Here's how the part is built. I have some questions about the finished solid (model axes, mm). Give positions to 0.01 mm unless a question says otherwise; leave off trailing zeros. Loops run counter-clockwise (first coordinate to the right, second up) from the corner with the lowest first, then second, coordinate; pieces in that order, holes last. Notation, with made-up numbers: M 23,70.5 L 42,70.5 A9 ccw 42,84.5 Z; hole C 24,36.5 d5. An arc over 180 degrees is marked long. Write item = value, one per line. Start each with the question number.
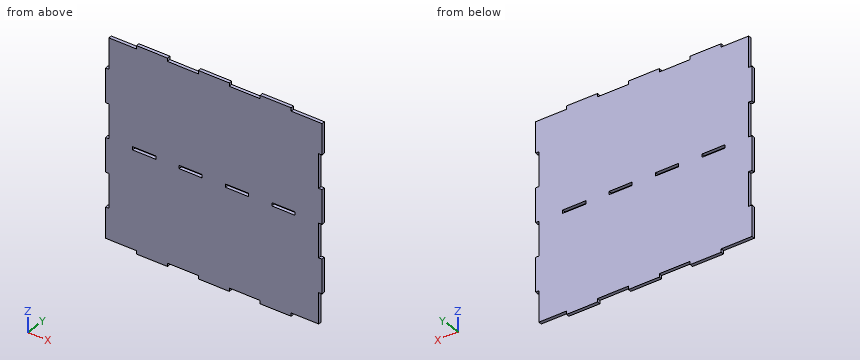
```python
from build123d import *

# Parameters (mm, degrees)
SKETCH1_W           = 21
SKETCH1_H           = 3
BOSS_EXTRUDE1_DEPTH = 3


with BuildPart() as part:
    # Sketch1 → Boss-Extrude1 (new body)
    with BuildSketch(Plane(origin=(0, 0, 0), x_dir=(1, 0, 0), z_dir=(0, 1, 0))):
        Polygon((-95, -62), (-95, -90), (-70, -90), (-70, -93), (-42, -93), (-42, -90), (-14, -90), (-14, -93), (14, -93), (14, -90), (42, -90), (42, -93), (70, -93), (70, -90), (98, -90), (98, -62), (95, -62), (95, -31), (98, -31), (98, 0), (95, 0), (95, 31), (98, 31), (98, 62), (95, 62), (95, 90), (70, 90), (70, 93), (42, 93), (42, 90), (14, 90), (14, 93), (-14, 93), (-14, 90), (-42, 90), (-42, 93), (-70, 93), (-70, 90), (-98, 90), (-98, 62), (-95, 62), (-95, 31), (-98, 31), (-98, 0), (-95, 0), (-95, -31), (-98, -31), (-98, -62), align=None)
        with Locations((-63, 0)):
            Rectangle(SKETCH1_W, SKETCH1_H, mode=Mode.SUBTRACT)
        with Locations((-21, 0)):
            Rectangle(SKETCH1_W, SKETCH1_H, mode=Mode.SUBTRACT)
        with Locations((21, 0)):
            Rectangle(SKETCH1_W, SKETCH1_H, mode=Mode.SUBTRACT)
        with Locations((63, 0)):
            Rectangle(SKETCH1_W, SKETCH1_H, mode=Mode.SUBTRACT)
    extrude(amount=BOSS_EXTRUDE1_DEPTH)


solid = part.part
```
Q1. Will these pins go through, and if not, where does the flat tip stop? pin 1 (1.5 mm diameter, centred on y = 1.5, z = 0.5, fed in from -X); pin 2 (1.5 mm diameter, centred on y = 2, z = 91, fed in from +X); pin 3 (0.9 mm diameter, centred on y = 1, z = 14.5, fed in from -X); pin 4 (1.5 mm diameter, centred on x = 96.5, y = 1, fed in from -Z).
Q2. If we section it at A-A, the plane x = 34.5: List the corners of the cut face in (y, z) for me, then the cut area to 3 significant figures.
Q3. If we section it at C-C, the plane y = 1.1: State how many separate pieces and enclosed holes the cut face has, then the cut area to 3 significant figures.
Q4. If we section it at B-B, the plane z = -72.5: List the corners of the cut face in (x, y) for me, then the cut area to 3 significant figures.
Q5. If I drill on line 1 along Z through (x, y) = (-23.5, 2.15); line 2 along Z through (x, y) = (-57.5, 2.7); line 3 along X through (y, z) = (2.8, -41), over which ranges is the centre line in solid material (lowest first)?
Resolved:
q1.pin_1 = -98
q1.pin_2 = 70
q1.pin_3 = -95
q1.pin_4 = -62
q2.outline = M 0,-90 L 3,-90 L 3,90 L 0,90 Z
q2.area = 540 mm²
q3.separate_pieces = 1
q3.enclosed_holes = 4
q3.area = 35,000 mm²
q4.outline = M -98,0 L 95,0 L 95,3 L -98,3 Z
q4.area = 579 mm²
q5.line_1 = -90 to -1.5, 1.5 to 90
q5.line_2 = -93 to -1.5, 1.5 to 93
q5.line_3 = -95 to 98
